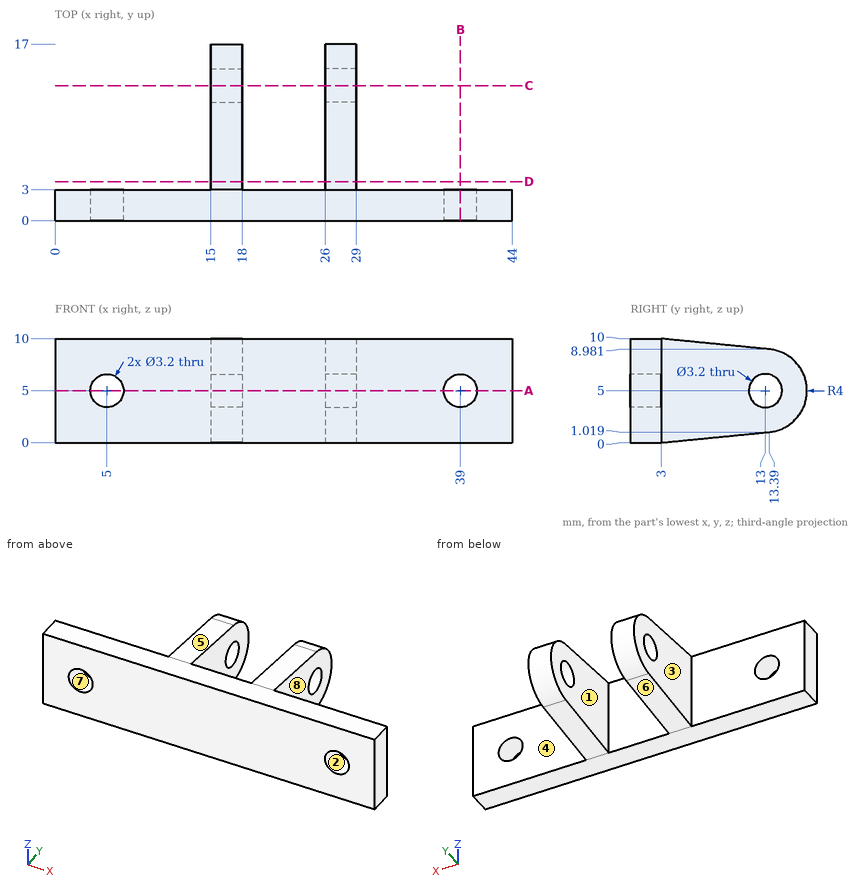
For this review, use the dimensioned drawing (mm, ordinates from the lowest corner) and the shaded views. A direction names the side the tool comes from. Coordinates: 2 decimals unless noted, no trailing zeros. Write each loop counter-clockwise with the first axis right and the second up, starting at its lowest first coordinate (ties: lowest second). Pieces come first, ordered by that corner, then holes. Notation, with made-up numbers: (-38, 6.5) - (13, 6.5) arc R25 ccw to (13, 18.5) - close; hole circle Ø6 at (24.5, -19). An arc over 180 degrees is marked (long way). Answer in a Markdown table with one row per item. Add a question column.
Q1. For the marked faces 1, 2, 3, 4 and 5, list the 3-axis set-ups (+Z, -Z, +X, -X, +Y, -Y) from which the entire face can be reached by the end or side of a thin tool; tool diameter is ignored.
Q2. To check wall thickness, follow line 1 along X through (y, z) = (13.5, 8.25); line 2 along Z through (x, y) = (39, 2); line 3 along X through (y, z) = (1.5, 5.5). State the ranges of each line that lie inside material, in increasing order. Write a range as from..to.
Q3. Consider section A-A on z = 5. Give the boundary of the cut face in (x, y).
Q4. Draft analysis for pull direction Z (two halves, no side actions). For the marked faces 6, 7 and 8, state which applies: +Z half, -Z half, draft (parallel to the pull), parting line (faces both ways), or undercut.
Q5. Clearance check with flat-ended pins moving along their axes: pin 1 (4 mm diameter, centred on y = 13, z = 5, fed in from -X); pin 2 (5 mm diameter, centred on y = 12.5, z = 6.5, fed in from +X); pin 3 (2.5 mm diameter, centred on x = 23.5, z = 5.5, fed in from +Y). State where each tip first meets the part, or that it passes through.
Q6. Consider section B-B on x = 39. Give the boundary of the cut face in (y, z).
Q7. Consider section C-C on y = 13. Give the boundary of the cut face in (x, z).
Q8. Consider section D-D on y = 3.75. Give the boundary of the cut face in (x, z).
Answers below:
| question | item | result |
|---|---|---|
| 1 | face 1 | +Z, -Z, +Y |
| 1 | face 2 | +Y, -Y |
| 1 | face 3 | +Z, -Z, -X, +Y |
| 1 | face 4 | +Z, -Z, +X, +Y |
| 1 | face 5 | +Z, +X, -X, +Y |
| 2 | line 1 | 15..18, 26..29 |
| 2 | line 2 | 0..3.4, 6.6..10 |
| 2 | line 3 | 0..3.48, 6.52..37.48, 40.52..44 |
| 3 | outline | (0, 0) - (3.4, 0) - (3.4, 3) - (0, 3) - close; (6.6, 0) - (37.4, 0) - (37.4, 3) - (29, 3) - (29, 11.4) - (26, 11.4) - (26, 3) - (18, 3) - (18, 11.4) - (15, 11.4) - (15, 3) - (6.6, 3) - close; (15, 14.6) - (18, 14.6) - (18, 17) - (15, 17) - close; (26, 14.6) - (29, 14.6) - (29, 17) - (26, 17) - close; (40.6, 0) - (44, 0) - (44, 3) - (40.6, 3) - close |
| 4 | face 6 | -Z half |
| 4 | face 7 | undercut |
| 4 | face 8 | draft |
| 5 | pin 1 | x = 15 |
| 5 | pin 2 | x = 29 |
| 5 | pin 3 | y = 3 |
| 6 | outline | (0, 0) - (3, 0) - (3, 3.4) - (0, 3.4) - close; (0, 6.6) - (3, 6.6) - (3, 10) - (0, 10) - close |
| 7 | outline | (15, 0.98) - (18, 0.98) - (18, 3.4) - (15, 3.4) - close; (15, 6.6) - (18, 6.6) - (18, 9.02) - (15, 9.02) - close; (26, 0.98) - (29, 0.98) - (29, 3.4) - (26, 3.4) - close; (26, 6.6) - (29, 6.6) - (29, 9.02) - (26, 9.02) - close |
| 8 | outline | (15, 0.07) - (18, 0.07) - (18, 9.93) - (15, 9.93) - close; (26, 0.07) - (29, 0.07) - (29, 9.93) - (26, 9.93) - close |
